from build123d import *

# Parameters (mm, degrees)
SALIENTE_EXTRUIR1_DEPTH = 40
CROQUIS4_R              = 2.25
CORTAR_EXTRUIR3_DEPTH   = 70.282032303
SALIENTE_EXTRUIR2_DEPTH = 20
CROQUIS8_R              = 4.15
CORTAR_EXTRUIR4_DEPTH   = 25
CROQUIS9_R              = 4.5
CORTAR_EXTRUIR6_DEPTH   = 20
CROQUIS9_4_R            = 4.5
CORTAR_EXTRUIR7_DEPTH   = 5.5
REDONDEO3_R             = 4
CORTAR_EXTRUIR8_DEPTH   = 1
CROQUIS11_R             = 5
SALIENTE_EXTRUIR3_DEPTH = 10


with BuildPart() as part:
    # Croquis1 → Saliente-Extruir1 (new body)
    with BuildSketch(Plane(origin=(0, 0, 0), x_dir=(1, 0, 0), z_dir=(0, 1, 0))):
        Polygon((0, 0), (40, 0), (40, 20), (20, 20), (20, 40), (0, 40), align=None)
    extrude(amount=SALIENTE_EXTRUIR1_DEPTH)

    # Croquis4 → Cortar-Extruir3 (cut, through all)
    with BuildSketch(Plane(origin=(0, 40, 0), x_dir=(1, 0, 0), z_dir=(0, 1, 0))):
        with Locations(Location((10, 30, 0), (0, 0, 270))):
            Circle(CROQUIS4_R)
        with Locations(Location((10, 10, 0), (0, 0, 270))):
            Circle(CROQUIS4_R)
    extrude(amount=-CORTAR_EXTRUIR3_DEPTH, mode=Mode.SUBTRACT)

    # Croquis5 → Saliente-Extruir2 (add)
    with BuildSketch(Plane.XY):
        with BuildLine():
            Line((0, 0), (0, 40))
            Line((0, 40), (-35, 40))
            ThreePointArc((-35, 40), (-55, 20), (-35, 0))
            Line((-35, 0), (0, 0))
        make_face()
    extrude(amount=-SALIENTE_EXTRUIR2_DEPTH)

    # Croquis8 → Cortar-Extruir4 (cut)
    with BuildSketch(Plane(origin=(40, 0, 0), x_dir=(0, 0, -1), z_dir=(1, 0, 0))):
        with Locations((10, 30)):
            Circle(CROQUIS8_R)
    extrude(amount=-CORTAR_EXTRUIR4_DEPTH, mode=Mode.SUBTRACT)

    # Croquis9 → Cortar-Extruir6 (cut)
    with BuildSketch(Plane(origin=(0, 0, -20), x_dir=(-1, 0, 0), z_dir=(0, 0, -1))):
        with Locations((29.5, 20)):
            Circle(CROQUIS9_R)
        with BuildLine():
            Line((12.9, 22.25), (15.1, 22.25))
            ThreePointArc((15.1, 22.25), (17.35, 20), (15.1, 17.75))
            Line((15.1, 17.75), (12.9, 17.75))
            ThreePointArc((12.9, 17.75), (10.65, 20), (12.9, 22.25))
        make_face()
        with BuildLine():
            Line((43.9, 17.75), (46.1, 17.75))
            ThreePointArc((46.1, 17.75), (48.35, 20), (46.1, 22.25))
            Line((46.1, 22.25), (43.9, 22.25))
            ThreePointArc((43.9, 22.25), (41.65, 20), (43.9, 17.75))
        make_face()
    extrude(amount=-CORTAR_EXTRUIR6_DEPTH, mode=Mode.SUBTRACT)

    # Croquis9_4 → Cortar-Extruir7 (cut)
    with BuildSketch(Plane(origin=(0, 0, -20), x_dir=(-1, 0, 0), z_dir=(0, 0, -1))):
        with BuildLine():
            Line((10.978313253, 25.472396189), (25.756024096, 30.661737402))
            ThreePointArc((25.756024096, 30.661737402), (29.5, 31.3), (33.243975904, 30.661737402))
            Line((33.243975904, 30.661737402), (48.021686747, 25.472396189))
            ThreePointArc((48.021686747, 25.472396189), (51.9, 20), (48.021686747, 14.527603811))
            Line((48.021686747, 14.527603811), (33.243975904, 9.338262598))
            ThreePointArc((33.243975904, 9.338262598), (29.5, 8.7), (25.756024096, 9.338262598))
            Line((25.756024096, 9.338262598), (10.978313253, 14.527603811))
            ThreePointArc((10.978313253, 14.527603811), (7.1, 20), (10.978313253, 25.472396189))
        make_face()
        with Locations((29.5, 20)):
            Circle(CROQUIS9_4_R, mode=Mode.SUBTRACT)
        with BuildLine():
            Line((12.9, 22.25), (15.1, 22.25))
            ThreePointArc((15.1, 22.25), (17.35, 20), (15.1, 17.75))
            Line((15.1, 17.75), (12.9, 17.75))
            ThreePointArc((12.9, 17.75), (10.65, 20), (12.9, 22.25))
        make_face(mode=Mode.SUBTRACT)
        with BuildLine():
            Line((43.9, 17.75), (46.1, 17.75))
            ThreePointArc((46.1, 17.75), (48.35, 20), (46.1, 22.25))
            Line((46.1, 22.25), (43.9, 22.25))
            ThreePointArc((43.9, 22.25), (41.65, 20), (43.9, 17.75))
        make_face(mode=Mode.SUBTRACT)
    extrude(amount=-CORTAR_EXTRUIR7_DEPTH, mode=Mode.SUBTRACT)

    # Redondeo3
    redondeo3_edges = [part.edges().sort_by_distance(p)[0] for p in [
        (0, 20, -40),
        (20, 20, -40),
        (20, 20, -20),
        (40, 20, -20),
        (40, 20, 0),
        (0, 20, -20),
    ]]
    fillet(redondeo3_edges, radius=REDONDEO3_R)

    # Croquis10 → Cortar-Extruir8 (cut)
    with BuildSketch(Plane(origin=(0, 40, 0), x_dir=(1, 0, 0), z_dir=(0, 1, 0))):
        Polygon((-10, 9.198317308), (-10, 10.307692308), (-4, 10.307692308), (-4, 9.769230769), (-9.384615385, 9.769230769), (-9.384615385, 8.846153846), align=None)
    extrude(amount=-CORTAR_EXTRUIR8_DEPTH, mode=Mode.SUBTRACT)

    # Croquis11 → Saliente-Extruir3 (add)
    with BuildSketch(Plane(origin=(0, 40, 0), x_dir=(1, 0, 0), z_dir=(0, 1, 0))):
        with BuildLine():
            Line((-16.985046875, 28.492523438), (-16.985046875, 20))
            Line((-16.985046875, 20), (-4, 20))
            ThreePointArc((-4, 20), (-1.171572875, 21.171572875), (0, 24))
            Line((0, 24), (0.123186534, 36.985046875))
            Line((0.123186534, 36.985046875), (-8.492523438, 36.985046875))
            ThreePointArc((-8.492523438, 36.985046875), (-14.49764435, 34.49764435), (-16.985046875, 28.492523438))
        make_face()
        with Locations(Location((-8.492523438, 28.492523438, 0), (0, 0, 270))):
            Circle(CROQUIS11_R, mode=Mode.SUBTRACT)
    extrude(amount=-SALIENTE_EXTRUIR3_DEPTH)


solid = part.part
Work out the finished part from the listing and answer in its coordinate system (mm). A direction names the side the tool comes from. Round coordinates to 2 decimals unless told otherwise and drop trailing zeros. Loops run counter-clockwise (first coordinate to the right, second up) from the corner with the lowest first, then second, coordinate; pieces in that order, holes last. Notation, with made-up numbers: M 73,0.5 L 128,0.5 A30 cw 128,38.5 Z; hole C 45,-31.75 d6. An arc over 180 degrees is marked long. One line per question, with ' | ' between items. Start each with the question number.
(1) A cutting plane is placed at B-B on z = -30. Write down the section's boundary in (x, y).
(2) Find the intervals of material crossed by line 1 (Y direction, x = -29.5, z = -6.75); line 2 (X direction, y = 27, z = -30); line 3 (X direction, y = 18, z = -24), in increasing order.
(3) A cutting plane is placed at A-A on y = 20. Give the number of separate pieces and of enclosed holes in the cut face, plus the area to 3 significant figures.
(4) A cutting plane is placed at D-D on y = 3.5. Write down the section's boundary in (x, z).
(5) A tool of negligible diameter and unlimited length cuts with its end or side. For faces 4 (the face through (11.52, 20.28, -11.66)), 5 (the face through (38.859, 20.28, -18.797)), 6 (the face through (-41.65, 20.05, -7.35)), 7 (the face through (-40.74, 11.97, -17.29)), 8 (the face through (-1.141, 15.21, -21.203)), from which of +Z, -Z, +X, -X, +Y, -Y can it reach the whole face along a straight path? Write none if from no direction.
(6) A cutting plane is placed at C-C on y = 37. Write down the section's boundary in (x, z).
(7) Flat-ended cylindrical pins translate along their axes: pin 1 Ø12 at (x, y) = (-18.5, 20) entering from -Z; pin 2 Ø3 at (x, z) = (-40, -5.5) entering from +Y; pin 3 Ø5 at (x, z) = (-4.5, -32) entering from -Y; pin 4 Ø8 at (x, z) = (24.5, -12) entering from -Y. Find the tip coordinate at first contact, or state that the pin passes through.
(8) For a pull along Y with two mould halves and no side action, classify faces 1 (the face through (-18.26, 28.03, -17.29)), 2 (the face through (-4.7, 30, -24.8)), 3 (the face through (20, 20, -30)) as released by +Y, released by -Y, zero draft, split by the parting line, or undercut.
Geometry check:
1) outline: M -16.85,30 L -13.26,30 L -13.26,40 L -16.85,40 Z; M -3.73,30 L 0,30 L 0,0 L 7.75,0 L 7.75,40 L -3.73,40 Z; M 12.25,0 L 20,0 L 20,40 L 12.25,40 Z
2) line 1: y = 0 to 15.5, 24.5 to 40 | line 2: x = 0 to 7.75, 12.25 to 20 | line 3: x = 0 to 20
3) separate pieces: 4 | enclosed holes: 2 | area: 1,690 mm²
4) outline: M -46.3,-20 L -4,-20 A4 cw 0,-24 L 0,-36 A4 ccw 4,-40 L 16,-40 A4 ccw 20,-36 L 20,-24 A4 cw 24,-20 L 36,-20 A4 ccw 40,-16 L 40,-4 A4 ccw 36,0 L -46.3,0 Z; hole C 10,-30 d4.5; hole C 10,-10 d4.5
5) face 4: +Y, -Y | face 5: -Z, +X, +Y, -Y | face 6: +Z, -Z | face 7: -Z | face 8: -Z, -X, -Y
6) outline: M -45.54,-20 L -16.99,-20 L -16.99,-28.49 A8.49 ccw -8.49,-36.99 L 0.12,-36.99 A4 ccw 4,-40 L 16,-40 A4 ccw 20,-36 L 20,-24 A4 cw 24,-20 L 36,-20 A4 ccw 40,-16 L 40,-4 A4 ccw 36,0 L -45.54,0 Z; hole C -8.49,-28.49 d10; hole C 10,-30 d4.5; hole C 10,-10 d4.5
7) pin 1: stops at z = -14.5 | pin 2: stops at y = 39.69 | pin 3: stops at y = 30 | pin 4: stops at y = 0
8) face 1: undercut | face 2: released by -Y | face 3: zero draft
